The listing builds one solid part. Answer for the finished solid, in the listing's coordinates (mm). A direction names the side the tool comes from. Round coordinates to 2 decimals unless told otherwise and drop trailing zeros. Loops run counter-clockwise (first coordinate to the right, second up) from the corner with the lowest first, then second, coordinate; pieces in that order, holes last. Notation, with made-up numbers: (-33.75, -35) -> (-13.75, -35) arc R16 cw to (-13.75, -20) -> close; hole circle Ø9 at (7, -29). An arc over 180 degrees is marked (long way). Answer in a Markdown table with one row per item. Add a question column.
```python
from build123d import *

# Parameters (mm, degrees)
SKETCH_2_W          = 16.4
SKETCH_2_H          = 19
SKETCH_2_W_2        = 4.3
SKETCH_2_H_2        = 13
EXTRUDE_1_DEPTH     = 2
SKETCH_3_W          = 8
SKETCH_3_H          = 2
EXTRUDE_2_DEPTH     = 12
SKETCH_10_W         = 3.8
SKETCH_10_H         = 19
EXTRUDE_4_DEPTH     = 1.7
CUT_EXTRUDE_START   = 1.7
SKETCH_9_R          = 0.375
CUT_EXTRUDE_2_DEPTH = 3.7
SKETCH_11_R         = 1.25
CUT_EXTRUDE_3_DEPTH = 26.294465798


with BuildPart() as part:
    # 草图2 → 凸台-拉伸1 (new body)
    with BuildSketch(Plane.XY):
        with Locations((-0.9, 0)):
            Rectangle(SKETCH_2_W, SKETCH_2_H)
        with Locations((-3.15, 0)):
            Rectangle(SKETCH_2_W_2, SKETCH_2_H_2, mode=Mode.SUBTRACT)
        with Locations((3.15, 0)):
            Rectangle(SKETCH_2_W_2, SKETCH_2_H_2, mode=Mode.SUBTRACT)
    extrude(amount=EXTRUDE_1_DEPTH)

    # 草图3 → 凸台-拉伸2 (add)
    with BuildSketch(Plane.XY.offset(2)):
        with Locations((3.3, 8.5)):
            Rectangle(SKETCH_3_W, SKETCH_3_H)
        with Locations((3.3, -8.5)):
            Rectangle(SKETCH_3_W, SKETCH_3_H)
    extrude(amount=EXTRUDE_2_DEPTH)

    # 草图10 → 凸台-拉伸4 (add)
    with BuildSketch(Plane.XY.offset(2)):
        with Locations((-7.2, 0)):
            Rectangle(SKETCH_10_W, SKETCH_10_H)
    extrude(amount=EXTRUDE_4_DEPTH)

    # 草图9 → 切除-拉伸2 (cut)
    with BuildSketch(Plane.XY.offset(2).offset(CUT_EXTRUDE_START)):
        with Locations((-7.2, 8)):
            Circle(SKETCH_9_R)
        with Locations((-7.2, -8)):
            Circle(SKETCH_9_R)
    extrude(amount=-CUT_EXTRUDE_2_DEPTH, mode=Mode.SUBTRACT)

    # 草图11 → 切除-拉伸3 (cut, through all)
    with BuildSketch(Plane.XZ.offset(9.5)):
        with Locations(Location((3.4, 10, 0), (0, 0, 270))):
            Circle(SKETCH_11_R)
    extrude(amount=-CUT_EXTRUDE_3_DEPTH, mode=Mode.SUBTRACT)


solid = part.part
```
Item 1: Section A-A, the plane x = -1.75 is taken. Write down the section's boundary in (y, z).
Item 2: Section D-D, the plane x = 3.4 is taken. Write down the section's boundary in (y, z).
Item 3: For faces 4 (the flat face through (3, 9, 14)), 5 (the flat face through (-3, -6.5, 1)), determine the directions among +Z, -Z, +X, -X, +Y, -Y from which every point of the face is accessible in a straight line to the end or side of a thin tool.
Item 4: Consider L1, parallel to Y at x = -7.2, z = 1.1 (3 decimals); L2, parallel to X at y = 2.75, z = 0.5; L3, parallel to X at y = 8.6, z = 10. Determine where each line is inside the solid, lowest interval first. Write a range as from..to.
Item 5: Flat-ended cylindrical pins translate along their axes: P1, Ø4, axis at x = 1, y = -1, coming from the +Z side; P2, Ø4, axis at x = -8, y = 2.5, coming from the +Z side; P3, Ø6, axis at y = 3.5, z = 6, coming from the +X side; P4, Ø1.5, axis at y = 5.5, z = 12.5, coming from the -X side. Find the tip coordinate at first contact, or state that the pin passes through.
Item 6: The mould has two halves that part along Y. Classify faces 1 (the flat face through (3, 6.5, 1)), 2 (the flat face through (3, 9.5, 5)), 3 (the flat face through (-0.7, -9, 8)): +Y half, -Y half, draft (parallel to the pull), parting line (faces both ways), or undercut.
Item 7: Section C-C, the plane y = 8 is taken. Write down the section's boundary in (x, z) (3 decimals), and give its area (3 significant figures).
Item 8: Section B-B, the plane z = 7.75 is taken. Write down the section's boundary in (x, y), and give its area (3 significant figures).
Here are the results:
| question | item | result |
|---|---|---|
| 1 | outline | (-9.5, 0) -> (-6.5, 0) -> (-6.5, 2) -> (-9.5, 2) -> close; (6.5, 0) -> (9.5, 0) -> (9.5, 2) -> (6.5, 2) -> close |
| 2 | outline | (-9.5, 0) -> (-6.5, 0) -> (-6.5, 2) -> (-7.5, 2) -> (-7.5, 8.75) -> (-9.5, 8.75) -> close; (-9.5, 11.25) -> (-7.5, 11.25) -> (-7.5, 14) -> (-9.5, 14) -> close; (6.5, 0) -> (9.5, 0) -> (9.5, 8.75) -> (7.5, 8.75) -> (7.5, 2) -> (6.5, 2) -> close; (7.5, 11.25) -> (9.5, 11.25) -> (9.5, 14) -> (7.5, 14) -> close |
| 3 | face 4 | +Z, +X, -X, +Y, -Y |
| 3 | face 5 | +Z, -Z |
| 4 | L1 | y = -9.5..-8.375, -7.625..7.625, 8.375..9.5 |
| 4 | L2 | x = -9.1..-5.3, -1..1, 5.3..7.3 |
| 4 | L3 | x = -0.7..2.15, 4.65..7.3 |
| 5 | P1 | stops at z = 2 |
| 5 | P2 | stops at z = 3.7 |
| 5 | P3 | stops at x = -5.3 |
| 5 | P4 | passes through |
| 6 | face 1 | undercut |
| 6 | face 2 | +Y half |
| 6 | face 3 | draft |
| 7 | outline | (-9.1, 0) -> (-7.575, 0) -> (-7.575, 3.7) -> (-9.1, 3.7) -> close; (-6.825, 0) -> (7.3, 0) -> (7.3, 14) -> (-0.7, 14) -> (-0.7, 2) -> (-5.3, 2) -> (-5.3, 3.7) -> (-6.825, 3.7) -> close; hole circle Ø2.5 at (3.4, 10) |
| 7 | area | 128 mm² |
| 8 | outline | (-0.7, -9.5) -> (7.3, -9.5) -> (7.3, -7.5) -> (-0.7, -7.5) -> close; (-0.7, 7.5) -> (7.3, 7.5) -> (7.3, 9.5) -> (-0.7, 9.5) -> close |
| 8 | area | 32.0 mm² |
